The listing builds one solid part. Answer for the finished solid, in the listing's coordinates (mm). Face numbers are marked on the shaded views. A direction names the side the tool comes from. Round coordinates to 2 decimals unless told otherwise and drop trailing zeros. Write each loop counter-clockwise with the first axis right and the second up, starting at its lowest first coordinate (ties: lowest second). Pieces come first, ordered by that corner, then holes.
Item 1: Find the intervals of material crossed by probe 1 along Z at (x, y) = (-62, -393.5); probe 2 along X at (y, z) = (-243.5, -124); probe 3 along X at (y, z) = (-388.5, 99), in increasing order.
Item 2: For a pull along Y with two mould halves and no side action, classify the marked faces 4, 5 and 6 as +Y half, -Y half, draft (parallel to the pull), parting line (faces both ways), or undercut.
Item 3: A tool of negligible diameter and unlimited length cuts with its end or side. For the marked faces 1, 2 and 3, from which of +Z, -Z, +X, -X, +Y, -Y can it reach the whole face along a straight path? Write none if from no direction.
Item 4: Each of these flat-tipped pins is pushed along its axis until it touches: pin 1 (6 mm diameter, centred on y = -231, z = -135, fed in from -X); pin 2 (20.5 mm diameter, centred on x = -98, y = -553.5, fed in from -Z); pin 3 (3 mm diameter, centred on x = 80.5, z = 131, fed in from +Y). Where does it stop, or does it pass through?
Item 5: Find section C-C on z = 36. Give the vertices of the cut face in (x, y), then the cut area to 3 significant figures.
Item 6: Find section B-B on y = -206.5. Give the vertices of the cut face in (x, z), then the cut area to 3 significant figures.
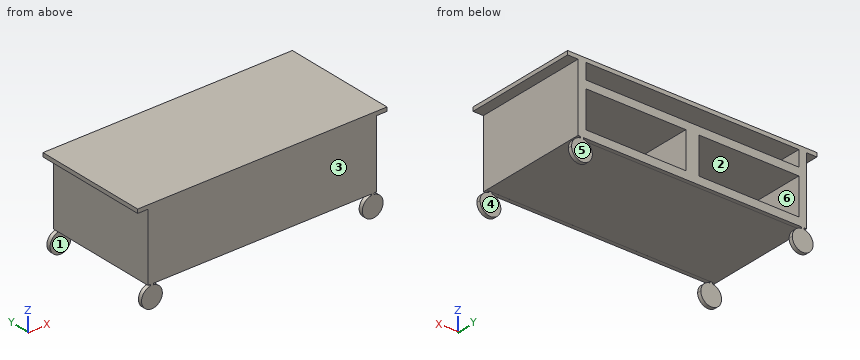
```python
from build123d import *

# Parameters (mm, degrees)
F0_W     = 63.5
F0_H     = 177.8
F1_DEPTH = 558.8
F4_DEPTH = 1412.24
F5_W     = 18.7272608757
F5_H     = 330.1743186474
F6_DEPTH = 1117.6


with BuildPart() as f1:
    # F0 (on Front) → F1 (new body)
    with BuildSketch(Plane.XZ):
        Polygon((-539.75, -165.1), (-533.4, -165.1), (-533.4, -148.0671259786), (-546.1, -148.0671259786), (-546.1, -165.1), align=None)
        Polygon((31.75, 50.8), (520.7, 50.8), (520.7, 88.9), (-520.7, 88.9), (-520.7, 50.8), (-31.75, 50.8), align=None)
        Polygon((-520.7, 165.1), (520.7, 165.1), (558.8, 165.1), (609.6, 165.1), (609.6, 184.15), (-609.6, 184.15), (-609.6, 165.1), (-558.8, 165.1), align=None)
        Polygon((533.4, -148.0671259786), (533.4, -165.1), (539.75, -165.1), (546.1, -165.1), (546.1, -148.0671259786), align=None)
        Polygon((-520.7, -165.1), (520.7, -165.1), (520.7, -127), (31.75, -127), (-31.75, -127), (-520.7, -127), align=None)
        with Locations((0, -38.1)):
            Rectangle(F0_W, F0_H)
        Polygon((520.7, -127), (520.7, -165.1), (533.4, -165.1), (533.4, -148.0671259786), (546.1, -148.0671259786), (546.1, -165.1), (558.8, -165.1), (558.8, 165.1), (520.7, 165.1), (520.7, 88.9), (520.7, 50.8), align=None)
        Polygon((-533.4, -165.1), (-520.7, -165.1), (-520.7, -127), (-520.7, 50.8), (-520.7, 88.9), (-520.7, 165.1), (-558.8, 165.1), (-558.8, -165.1), (-546.1, -165.1), (-546.1, -148.0671259786), (-533.4, -148.0671259786), align=None)
        with BuildLine():
            Line((-539.75, -171.45), (-539.75, -165.1))
            Line((-539.75, -165.1), (-546.1, -165.1))
            Line((-546.1, -165.1), (-546.1, -171.8484375242))
            ThreePointArc((-546.1, -171.8484375242), (-542.9312439572, -171.5497072308), (-539.75, -171.45))
        make_face()
        with BuildLine():
            Line((-533.4, -171.8484375242), (-533.4, -165.1))
            Line((-533.4, -165.1), (-539.75, -165.1))
            Line((-539.75, -165.1), (-539.75, -171.45))
            ThreePointArc((-539.75, -171.45), (-536.5687560428, -171.5497072308), (-533.4, -171.8484375242))
        make_face()
        with BuildLine():
            Line((-533.4, -182.1328740214), (-533.4, -171.8484375242))
            ThreePointArc((-533.4, -171.8484375242), (-536.5687560428, -171.5497072308), (-539.75, -171.45))
            Line((-539.75, -171.45), (-539.75, -182.1328740214))
            Line((-539.75, -182.1328740214), (-533.4, -182.1328740214))
        make_face()
        with BuildLine():
            Line((-539.75, -182.1328740214), (-539.75, -171.45))
            ThreePointArc((-539.75, -171.45), (-542.9312439572, -171.5497072308), (-546.1, -171.8484375242))
            Line((-546.1, -171.8484375242), (-546.1, -182.1328740214))
            Line((-546.1, -182.1328740214), (-539.75, -182.1328740214))
        make_face()
        with BuildLine():
            ThreePointArc((-488.95, -222.25), (-501.65, -188.6489583495), (-533.4, -171.8484375242))
            Line((-533.4, -171.8484375242), (-533.4, -182.1328740214))
            Line((-533.4, -182.1328740214), (-539.75, -182.1328740214))
            Line((-539.75, -182.1328740214), (-546.1, -182.1328740214))
            Line((-546.1, -182.1328740214), (-546.1, -171.8484375242))
            ThreePointArc((-546.1, -171.8484375242), (-573.3510416505, -260.35), (-488.95, -222.25))
        make_face()
        with BuildLine():
            Line((539.75, -165.1), (533.4, -165.1))
            Line((533.4, -165.1), (533.4, -171.8484375242))
            ThreePointArc((533.4, -171.8484375242), (536.5687560428, -171.5497072308), (539.75, -171.45))
            Line((539.75, -171.45), (539.75, -165.1))
        make_face()
        with BuildLine():
            ThreePointArc((539.75, -171.45), (536.5687560428, -171.5497072308), (533.4, -171.8484375242))
            Line((533.4, -171.8484375242), (533.4, -182.1328740214))
            Line((533.4, -182.1328740214), (539.75, -182.1328740214))
            Line((539.75, -182.1328740214), (539.75, -171.45))
        make_face()
        with BuildLine():
            Line((546.1, -165.1), (539.75, -165.1))
            Line((539.75, -165.1), (539.75, -171.45))
            ThreePointArc((539.75, -171.45), (542.9312439572, -171.5497072308), (546.1, -171.8484375242))
            Line((546.1, -171.8484375242), (546.1, -165.1))
        make_face()
        with BuildLine():
            ThreePointArc((546.1, -171.8484375242), (542.9312439572, -171.5497072308), (539.75, -171.45))
            Line((539.75, -171.45), (539.75, -182.1328740214))
            Line((539.75, -182.1328740214), (546.1, -182.1328740214))
            Line((546.1, -182.1328740214), (546.1, -171.8484375242))
        make_face()
        with BuildLine():
            Line((533.4, -182.1328740214), (533.4, -171.8484375242))
            ThreePointArc((533.4, -171.8484375242), (506.1489583495, -260.35), (590.55, -222.25))
            ThreePointArc((590.55, -222.25), (577.85, -188.6489583495), (546.1, -171.8484375242))
            Line((546.1, -171.8484375242), (546.1, -182.1328740214))
            Line((546.1, -182.1328740214), (539.75, -182.1328740214))
            Line((539.75, -182.1328740214), (533.4, -182.1328740214))
        make_face()
    extrude(amount=F1_DEPTH)

    # F3 (on offset) → F4 (cut)
    with BuildSketch(Plane(origin=(-762, 0, 0), x_dir=(0, -1, 0), z_dir=(-1, 0, 0))):
        Polygon((540.0727391243, -165.0743186474), (19.05, -165.0743186474), (19.05, -171.5670526028), (19.05, -304.82172966), (540.0727391243, -304.82172966), (540.0727391243, -173.7104952335), align=None)
    extrude(amount=-F4_DEPTH, mode=Mode.SUBTRACT)

    # F5 (on face) → F6 (join)
    with BuildSketch(Plane.YZ.offset(558.8)):
        with Locations((-549.4363695621, 0.0128406763)):
            Rectangle(F5_W, F5_H)
    extrude(amount=-F6_DEPTH)


solid = f1.part
```
Check values:
1. probe 1: z = -165.07 to -127, 50.8 to 88.9, 165.1 to 184.15
1. probe 2: x = -558.8 to -520.7, -31.75 to 31.75, 520.7 to 558.8
1. probe 3: x = -558.8 to -520.7, 520.7 to 558.8
2. face 4: undercut
2. face 5: +Y half
2. face 6: draft
3. face 1: -Z, +X, -X
3. face 2: +Y
3. face 3: +Z, -Z, +X, -X, -Y
4. pin 1: stops at x = -558.8
4. pin 2: stops at z = -165.1
4. pin 3: stops at y = -540.07
5. outline: (-558.8, -558.8) - (558.8, -558.8) - (558.8, 0) - (520.7, 0) - (520.7, -540.07) - (31.75, -540.07) - (31.75, 0) - (-31.75, 0) - (-31.75, -540.07) - (-520.7, -540.07) - (-520.7, 0) - (-558.8, 0) - close
5. area: 96,400 mm2
6. outline: (-609.6, 165.1) - (-558.8, 165.1) - (-558.8, -165.07) - (558.8, -165.07) - (558.8, 165.1) - (609.6, 165.1) - (609.6, 184.15) - (-609.6, 184.15) - close; hole (-520.7, -127) - (-31.75, -127) - (-31.75, 50.8) - (-520.7, 50.8) - close; hole (-520.7, 88.9) - (520.7, 88.9) - (520.7, 165.1) - (-520.7, 165.1) - close; hole (31.75, -127) - (520.7, -127) - (520.7, 50.8) - (31.75, 50.8) - close
6. area: 139,000 mm2
